For this review, take the finished solid that the model builds, in its own axes (mm). Face numbers are marked on the shaded views. A direction names the side the tool comes from. Round coordinates to 2 decimals unless told otherwise and drop trailing zeros. Order: outer loops, then holes, each group sorted by start corner. A loop starts at its lowest first (then second) coordinate and runs counter-clockwise, first axis right, second up. Notation, with made-up numbers: M 31,-20.5 L 73,-20.5 A19 ccw 73,15.5 Z; hole C 5,37.5 d10. An arc over 180 degrees is marked long. Put each result on its own line as item: value.
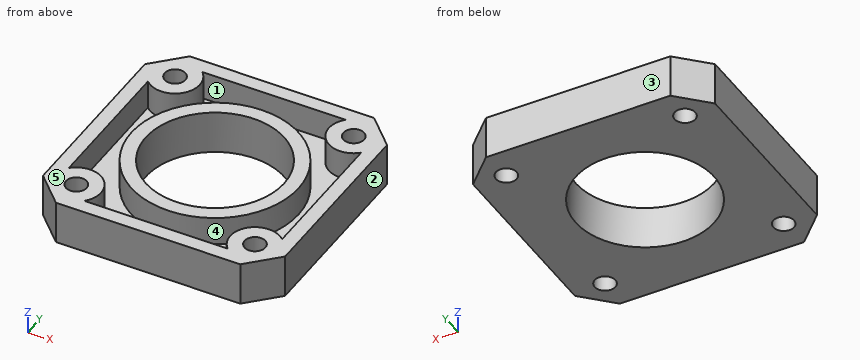
from build123d import *

# Parameters (mm, degrees)
F0_W     = 42
F0_H     = 42
F0_R     = 1.8
F0_R_2   = 12
F1_DEPTH = 7.5
F2_SIZE  = 5
F3_T     = -2.5


with BuildPart() as f1:
    # F0 (on Top) → F1 (new body)
    with BuildSketch(Plane.XY):
        Rectangle(F0_W, F0_H)
        with Locations((-15.5, -15.5)):
            Circle(F0_R, mode=Mode.SUBTRACT)
        with Locations((15.5, -15.5)):
            Circle(F0_R, mode=Mode.SUBTRACT)
        with Locations((-15.5, 15.5)):
            Circle(F0_R, mode=Mode.SUBTRACT)
        Circle(F0_R_2, mode=Mode.SUBTRACT)
        with Locations((15.5, 15.5)):
            Circle(F0_R, mode=Mode.SUBTRACT)
    extrude(amount=F1_DEPTH)

    # F2
    f2_edges = [f1.edges().sort_by_distance(p)[0] for p in [
        (21, -21, 3.75),
        (21, 21, 3.75),
        (-21, -21, 3.75),
        (-21, 21, 3.75),
    ]]
    chamfer(f2_edges, length=F2_SIZE)

    # F3
    f3_openings = [f1.faces().sort_by_distance(p)[0] for p in [
        (20.40603, 0, 7.5),
    ]]
    offset(amount=F3_T, openings=f3_openings)


solid = f1.part
(1) Add section C-C on y = 15.5. Give the boundary of the cut face in (x, z).
A:
outline: M -21,0 L -17.3,0 L -17.3,7.5 L -21,7.5 Z; M -13.7,0 L 13.7,0 L 13.7,7.5 L 11.2,7.5 L 11.2,2.5 L -11.2,2.5 L -11.2,7.5 L -13.7,7.5 Z; M 17.3,0 L 21,0 L 21,7.5 L 17.3,7.5 Z
(2) To check wall thickness, follow L1, parallel to Y at x = 15.5, z = 2.75; L2, parallel to Y at x = 0, z = 3.75; L3, parallel to Y at x = -13, z = 2.75. State the ranges of each line that lie inside material, in increasing order.
A:
L1: y = -21 to -17.3, -13.7 to -11.2, 11.2 to 13.7, 17.3 to 21
L2: y = -21 to -18.5, -14.5 to -12, 12 to 14.5, 18.5 to 21
L3: y = -21 to -12, -6.42 to 6.42, 12 to 21
(3) Insertion check: pin 1 Ø3 at (x, y) = (15.5, -15.5) entering from -Z. The pin has a flat end and moves straight along its axis. Give the tip position at first contact, or say it passes through.
A:
pin 1: passes through
(4) Draft analysis for pull direction X (two halves, no side actions). For the marked faces 1, 2 and 3, state which applies: released by +X, released by -X, zero draft, split by the parting line, or undercut.
A:
face 1: undercut
face 2: released by +X
face 3: zero draft
(5) Add section A-A on z = 4.5. Give the boundary of the cut face in (x, y), then the cut area to 3 significant figures.
A:
outline: M -21,-16 L -16,-21 L 16,-21 L 21,-16 L 21,16 L 16,21 L -16,21 L -21,16 Z; C 0,0 d29; hole M -18.5,-12.42 A4.3 cw -12.42,-18.5 L 12.42,-18.5 A4.3 cw 18.5,-12.42 L 18.5,12.42 A4.3 cw 12.42,18.5 L -12.42,18.5 A4.3 cw -18.5,12.42 Z; hole C -15.5,-15.5 d3.6; hole C -15.5,15.5 d3.6; hole C 0,0 d24; hole C 15.5,-15.5 d3.6; hole C 15.5,15.5 d3.6
area: 701 mm2
(6) For the marked faces 4 and 5, list the 3-axis set-ups (+Z, -Z, +X, -X, +Y, -Y) from which the entire face can be reached by the end or side of a thin tool; tool diameter is ignored.
A:
face 4: +Z
face 5: +Z, +X, -X, +Y, -Y
(7) Add section B-B on x = 0. Give the boundary of the cut face in (y, z), then the cut area to 3 significant figures.
A:
outline: M -21,0 L -12,0 L -12,7.5 L -14.5,7.5 L -14.5,2.5 L -18.5,2.5 L -18.5,7.5 L -21,7.5 Z; M 12,0 L 21,0 L 21,7.5 L 18.5,7.5 L 18.5,2.5 L 14.5,2.5 L 14.5,7.5 L 12,7.5 Z
area: 95.0 mm2
